Autodesk Inventor part; units mm, degrees
ref_plane "YZ Plane" through (0, 0, 0) normal (1, 0, 0) x (0, 1, 0)
ref_plane "XZ Plane" through (0, 0, 0) normal (0, 1, 0) x (-1, 0, 0)
ref_plane "XY Plane" through (0, 0, 0) normal (0, 0, 1) x (1, 0, 0)
sketch "Sketch4" plane through (0, 0, 0) normal (0, 1, 0) x (-1, 0, 0)
  circle A0 centre (0, 0) radius 38.735
  circle A1 centre (0, 0) radius 50.8
  dimension "d9" = 77.47
  dimension "d10" = 101.6
extrude "Extrusion2" add sketch "Sketch4" along normal blind 6.35
sketch "Sketch5" plane through (0, 6.35, 0) normal (0, 1, 0) x (1, 0, 0)
  circle A0 centre (0, -44.45) radius 2.667
  circle A1 centre (38.4948, -22.225) radius 2.667
  circle A2 centre (38.4948, 22.225) radius 2.667
  circle A3 centre (0, 44.45) radius 2.667
  circle A4 centre (-38.4948, 22.225) radius 2.667
  circle A5 centre (-38.4948, -22.225) radius 2.667
  point P0 (0, 0)
  dimension "d13" = 5.334
  dimension "d16" = 360
extrude "Extrusion3" cut sketch "Sketch5" against normal blind 6.35
sketch "Sketch7" plane through (0, 6.35, 0) normal (0, 1, 0) x (1, 0, 0)
  line L0 (50.8, 12.7) -> (81.788, 12.7)
  line L1 (81.788, 12.7) -> (81.788, -12.7)
  line L2 (81.788, -12.7) -> (50.8, -12.7)
  line L3 (50.8, -12.7) -> (50.8, 12.7)
  line L4 (-50.8, 12.7) -> (-81.788, 12.7)
  line L5 (-81.788, 12.7) -> (-81.788, -12.7)
  line L6 (-81.788, -12.7) -> (-50.8, -12.7)
  line L7 (-50.8, -12.7) -> (-50.8, 12.7)
  point P0 (0, 0)
  dimension "d50" = 30.988
  dimension "d51" = 25.4
  dimension "d52" = 30.988
extrude "Extrusion4" add sketch "Sketch7" against normal blind 6.35
sketch "Sketch8" plane through (0, 6.35, 0) normal (0, 1, 0) x (1, 0, 0)
  line L0 (-123.5202, 12.7) -> (-50.8, 12.7)
  line L1 (-60.9386, 12.7) -> (-45.3133, 12.7)
  line L2 (-45.3133, 12.7) -> (-45.3133, -12.7)
  line L3 (-45.3133, -12.7) -> (-60.9386, -12.7)
  line L4 (-60.9386, -12.7) -> (-60.9386, 12.7)
  line L5 (57.1886, 12.7) -> (43.7508, 12.7)
  line L6 (43.7508, 12.7) -> (43.7508, -12.7)
  line L7 (43.7508, -12.7) -> (57.1886, -12.7)
  line L8 (57.1886, -12.7) -> (57.1886, 12.7)
  point P0 (0, 0)
extrude "Extrusion5" add sketch "Sketch8" against normal blind 6.35
sketch "Sketch9" plane through (0, 6.35, 0) normal (0, 1, 0) x (1, 0, 0)
  line L0 (111.76, 12.7) -> (111.76, -12.7)
  line L1 (81.788, 12.7) -> (81.788, -12.7)
  circle A0 centre (81.788, 0) radius 12.7
  line L2 (-81.788, 12.7) -> (-81.788, -12.7)
  circle A1 centre (-81.788, 0) radius 12.7
  point P0 (0, 0)
  point P1 (-111.7602, 0)
  point P2 (-111.76, -12.7)
extrude "Extrusion6" add sketch "Sketch9" against normal blind 6.35
sketch "Sketch10" plane through (0, 6.35, 0) normal (0, 1, 0) x (1, 0, 0)
  circle A0 centre (81.28, 0) radius 3.175
  circle A1 centre (91.3638, 0) radius 1.27
  circle A2 centre (76.2381, 8.7328) radius 1.27
  circle A3 centre (76.2381, -8.7328) radius 1.27
  circle A4 centre (-81.28, 0) radius 3.175
  circle A5 centre (-91.3638, 0) radius 1.27
  circle A6 centre (-76.2381, -8.7328) radius 1.27
  circle A7 centre (-76.2381, 8.7328) radius 1.27
  point P0 (0, 0)
  dimension "d53" = 6.35
  dimension "d54" = 2.54
  dimension "d57" = 360
  dimension "d59" = 6.35
  dimension "d60" = 2.54
  dimension "d63" = 360
extrude "Extrusion7" cut sketch "Sketch10" against normal blind 6.35
properties part number "middle plate"
Model file for the job. Use its own axes, mm. A direction names the side the tool comes from. Give positions to 0.01 mm unless a question says otherwise; leave off trailing zeros. Loops run counter-clockwise (first coordinate to the right, second up) from the corner with the lowest first, then second, coordinate; pieces in that order, holes last. Notation, with made-up numbers: (-36, 17) - (9, 17) arc R23 ccw to (9, 37) - close; hole circle Ø8 at (16.5, 75). An arc over 180 degrees is marked (long way). One line per item, written item: value. Start each with the question number.
1. Slice it at D-D (x = -53). List the corners of the cut face in (y, z), plus the area to 3 significant figures.
2. Which spindle directions (+Z, -Z, +X, -X, +Y, -Y) get a long thin tool onto all of the face, cutting with end or side? Do faces 4 (the flat face through (-65, 3, 12.7)), 5 (the flat face through (-28, 6.35, -27)), 6 (the flat face through (-66, 3, -12.7)). Say none if no direction does.
3. Probe L1, parallel to Z at x = -76, y = 4.25; L2, parallel to X at y = 1.25, z = -20.5; L3, parallel to X at y = 3.75, z = 22. List the from-to ranges inside material, lowest first. Write a range as from..to.
4. Slice it at C-C (y = 4.5). Give the number of separate pieces and of enclosed holes in the cut face, plus the area to 3 significant figures.
5. Slice it at A-A (z = -30.5). List the corners of the cut face in (x, y) (3 decimals).
6. Pin check, flat tips, straight feed: pin 1 (8.5 mm diameter, centred on x = -38.49, z = 22.22, fed in from +Y); pin 2 (2 mm diameter, centred on y = 1, z = -4, fed in from +X); pin 3 (1.5 mm diameter, centred on x = 5, y = 0.5, fed in from +Z). Stop position of each tip, or through.
7. Pull direction X, two halves, no side cores. Call faces 1 (the flat face through (66, 3, -12.7)), 2 (the cylindrical face through (-78.25, 3.22, -0.95)), 3 (the cylindrical face through (-0.94, 3.13, -50.79)): pulls with the +X half, pulls with the -X half, needs draft (parallel to the pull), parting line crosses it, or undercut.
8. Slice it at B-B (x = 6). List the corners of the cut face in (y, z), plus the area to 3 significant figures.
Solution:
1. outline: (0, -12.7) - (6.35, -12.7) - (6.35, 12.7) - (0, 12.7) - close
1. area: 161 mm^2
2. face 4: +Z, -X, +Y, -Y
2. face 5: +Z, -Z, +X, -X, +Y
2. face 6: -Z, -X, +Y, -Y
3. L1: z = -12.7..-9.98, -7.49..7.49, 9.98..12.7
3. L2: x = -46.48..-40.53, -36.46..-32.87, 32.87..36.46, 40.53..46.48
3. L3: x = -45.79..-41.15, -35.84..-31.88, 31.88..35.84, 41.15..45.79
4. separate pieces: 1
4. enclosed holes: 15
4. area: 5,270 mm^2
5. outline: (-40.625, 0) - (-23.878, 0) - (-23.878, 6.35) - (-40.625, 6.35) - close; (23.878, 0) - (40.625, 0) - (40.625, 6.35) - (23.878, 6.35) - close
6. pin 1: stops at y = 6.35
6. pin 2: stops at x = 94.13
6. pin 3: stops at z = 50.62
7. face 1: needs draft
7. face 2: undercut
7. face 3: parting line crosses it
8. outline: (0, -50.44) - (6.35, -50.44) - (6.35, -38.27) - (0, -38.27) - close; (0, 38.27) - (6.35, 38.27) - (6.35, 50.44) - (0, 50.44) - close
8. area: 155 mm^2
